For this review, take the finished solid that the model builds, in its own axes (mm). A direction names the side the tool comes from. Round coordinates to 2 decimals unless told otherwise and drop trailing zeros. Order: outer loops, then holes, each group sorted by start corner. A loop starts at its lowest first (then second) coordinate and runs counter-clockwise, first axis right, second up. Notation, with made-up numbers: (55, -15.5) -> (96, -15.5) arc R35 ccw to (96, 23.5) -> close; hole circle Ø7 at (-20.5, 57.5). An arc over 180 degrees is marked (long way). Use a Markdown table: item, result. Add a question column.
1) Draft analysis for pull direction Y (two halves, no side actions). For faces 1 (the face through (27.822, 16, 12)), 2 (the face through (-53.228, -27.144, 28.574)), 3 (the face through (-40, 35, 3)), state which applies: pulls with the +Y half, pulls with the -Y half, needs draft (parallel to the pull), parting line crosses it, or undercut.
2) Wall thickness on line 1 along Y through (x, z) = (-40, 22); line 2 along X through (y, z) = (49.5, 9.5); line 3 along X through (y, z) = (-9.5, 9.5): over which ranges is each line inside the solid? List them lowest first. Write a range as [from, to].
3) Clearance check with a flat-ended pin moving along its axis: P1, Ø6, axis at x = -75.5, y = 1, coming from the +Z side. State where the tip first meets the part, or that it passes through.
4) Machinability: for faces 4 (the face through (-51.128, 59.849, 28.574)), 5 (the face through (0.609, 10.735, 14.832)), which of the approach directions +Z, -Z, +X, -X, +Y, -Y give a long, thin tool a straight path to every point of the face, cutting with its end or side? Answer none if there is none.
5) Consider section A-A (z = 12). State the section outline as (x, y) points, plus the area to 3 significant figures.
```python
from build123d import *

# Parameters (mm, degrees)
F0_W     = 160
F0_H     = 90
F0_R     = 30
F0_R_2   = 13.5
F0_R_3   = 17
F0_R_4   = 18.5
F1_DEPTH = 30
F2_DEPTH = 3
F3_R     = 5
F4_R     = 5


# Not quite as in the source:
# - a fillet or chamfer that OpenCascade refuses, or shapes differently, is made with other operations: its cross-section is extruded or revolved along the edge and cut away or added


with BuildPart() as f1:
    # F0 (on Top) → F1 (new body)
    with BuildSketch(Plane.XY):
        with Locations((-52.1784374716, 16.3527858257)):
            Rectangle(F0_W, F0_H)
        with Locations((-94.1784374716, 15.4254203662)):
            Circle(F0_R, mode=Mode.SUBTRACT)
        with Locations((-39.6653786302, -7.1472141743)):
            Circle(F0_R_2, mode=Mode.SUBTRACT)
        with Locations((2.8215625284, -6.1201333007)):
            Circle(F0_R_3, mode=Mode.SUBTRACT)
        with Locations((-39.6653786302, 34.8527858257)):
            Circle(F0_R_4, mode=Mode.SUBTRACT)
        with Locations((2.8215625284, 35.9062709907)):
            Circle(F0_R_3, mode=Mode.SUBTRACT)
    extrude(amount=F1_DEPTH)

    # F0 (on Top) → F2 (join)
    with BuildSketch(Plane.XY):
        with Locations((-52.1784374716, 16.3527858257)):
            Rectangle(F0_W, F0_H)
        with Locations((-94.1784374716, 15.4254203662)):
            Circle(F0_R, mode=Mode.SUBTRACT)
        with Locations((-39.6653786302, -7.1472141743)):
            Circle(F0_R_2, mode=Mode.SUBTRACT)
        with Locations((2.8215625284, -6.1201333007)):
            Circle(F0_R_3, mode=Mode.SUBTRACT)
        with Locations((-39.6653786302, 34.8527858257)):
            Circle(F0_R_4, mode=Mode.SUBTRACT)
        with Locations((2.8215625284, 35.9062709907)):
            Circle(F0_R_3, mode=Mode.SUBTRACT)
        with Locations((-94.1784374716, 15.4254203662)):
            Circle(F0_R)
        with Locations((-39.6653786302, -7.1472141743)):
            Circle(F0_R_2)
        with Locations((2.8215625284, -6.1201333007)):
            Circle(F0_R_3)
        with Locations((2.8215625284, 35.9062709907)):
            Circle(F0_R_3)
        with Locations((-39.6653786302, 34.8527858257)):
            Circle(F0_R_4)
    extrude(amount=F2_DEPTH)

    # F3
    f3_edges = [f1.edges().sort_by_distance(p)[0] for p in [
        (27.821563, 61.352786, 15),
        (27.821563, -28.647214, 15),
        (-132.178437, -28.647214, 15),
        (-132.178437, 61.352786, 15),
    ]]
    fillet(f3_edges, radius=F3_R)

    # F4
    f4_edges = [f1.edges().sort_by_distance(p)[0] for p in [
        (-52.178437, 61.352786, 30),
        (27.821563, 16.352786, 30),
        (-52.178437, -28.647214, 30),
        (-132.178437, 16.352786, 30),
        (26.357096, -27.182748, 30),
        (26.357096, 59.88832, 30),
        (-130.713971, -27.182748, 30),
        (-130.713971, 59.88832, 30),
    ]]
    fillet(f4_edges, radius=F4_R)

    # F5: chamfer of 3 on 5 edges, made by hand

    # F5_s1 → F5_t2 (revolve, cut)
    with BuildSketch(Plane.XZ.offset(-15.4254203662)):
        Polygon((-61.1784374716, 30), (-64.1784374716, 27), (-64.1784374716, 30), align=None)
    revolve(axis=Axis((-94.1784374716, 15.4254203662, 30), (0, 0, 1)), mode=Mode.SUBTRACT)

    # F5_s3 → F5_t4 (revolve, cut)
    with BuildSketch(Plane.XZ.offset(-34.8527858257)):
        Polygon((-18.1653786302, 30), (-21.1653786302, 27), (-21.1653786302, 30), align=None)
    revolve(axis=Axis((-39.6653786302, 34.8527858257, 30), (0, 0, 1)), mode=Mode.SUBTRACT)

    # F5_s5 → F5_t6 (revolve, cut)
    with BuildSketch(Plane.XZ.offset(-35.9062709907)):
        Polygon((22.8215625284, 30), (19.8215625284, 27), (19.8215625284, 30), align=None)
    revolve(axis=Axis((2.8215625284, 35.9062709907, 30), (0, 0, 1)), mode=Mode.SUBTRACT)

    # F5_s7 → F5_t8 (revolve, cut)
    with BuildSketch(Plane.XZ.offset(6.1201333007)):
        Polygon((22.8215625284, 30), (19.8215625284, 27), (19.8215625284, 30), align=None)
    revolve(axis=Axis((2.8215625284, -6.1201333007, 30), (0, 0, 1)), mode=Mode.SUBTRACT)

    # F5_s9 → F5_t10 (revolve, cut)
    with BuildSketch(Plane.XZ.offset(7.1472141743)):
        Polygon((-23.1653786302, 30), (-26.1653786302, 27), (-26.1653786302, 30), align=None)
    revolve(axis=Axis((-39.6653786302, -7.1472141743, 30), (0, 0, 1)), mode=Mode.SUBTRACT)


solid = f1.part
```
Results list:
| question | item | result |
|---|---|---|
| 1 | face 1 | needs draft |
| 1 | face 2 | pulls with the -Y half |
| 1 | face 3 | undercut |
| 2 | line 1 | [-28.65, -20.64], [6.35, 16.36], [53.35, 61.35] |
| 2 | line 2 | [-132.18, -50.97], [-28.36, -7.39], [13.03, 27.82] |
| 2 | line 3 | [-132.18, -110.87], [-77.48, -52.96], [-26.37, -13.84], [19.48, 27.82] |
| 3 | P1 | z = 3 |
| 4 | face 4 | +Z, +X, -X, +Y |
| 4 | face 5 | +Z |
| 5 | outline | (-132.18, -23.65) arc R5 ccw to (-127.18, -28.65) -> (22.82, -28.65) arc R5 ccw to (27.82, -23.65) -> (27.82, 56.35) arc R5 ccw to (22.82, 61.35) -> (-127.18, 61.35) arc R5 ccw to (-132.18, 56.35) -> close; hole circle Ø60 at (-94.18, 15.43); hole circle Ø37 at (-39.67, 34.85); hole circle Ø27 at (-39.67, -7.15); hole circle Ø34 at (2.82, -6.12); hole circle Ø34 at (2.82, 35.91) |
| 5 | area | 8,090 mm2 |
